Autodesk Fusion 360 part; units mm, degrees
sketch "Sketch1" plane through (0, 0, 0) normal (0, 0, 1) x (1, 0, 0)
  circle A0 centre (18.5, 32.0429) radius 7.5
  circle A1 centre (18.5, -32.0429) radius 7.5
  line L0 (0, 0) -> (80.5902, 0) construction
  line L1 (0, 0) -> (18.5, 32.0429) construction
  arc A2 (14.75, 25.5477) -> (14.75, -25.5477) centre (0, 0) ccw
  arc A3 (13.1121, 37.2602) -> (13.1121, -37.2602) centre (0, 0) ccw
  line L2 (-25.6953, 30) -> (-95.6953, 30)
  line L3 (-95.6953, -30) -> (-25.6953, -30)
  line L4 (0, 0) -> (-230.6084, 0) construction
  circle A4 centre (18.5, 32.0429) radius 3.5
  circle A5 centre (18.5, -32.0429) radius 3.5
  line L5 (-105.6953, 20) -> (-105.6953, -20)
  arc A6 (-95.6953, 30) -> (-105.6953, 20) centre (-95.6953, 20) ccw
  arc A7 (-105.6953, -20) -> (-95.6953, -30) centre (-95.6953, -20) ccw
  circle A8 centre (-95.6953, 20) radius 2.5
  circle A9 centre (-95.6953, -20) radius 2.5
  circle A10 centre (-45.6953, -20) radius 2.5
  circle A11 centre (-45.6953, 20) radius 2.5
  circle A12 centre (-70.6953, 20) radius 2.5
  circle A13 centre (-70.6953, -20) radius 2.5
  point P0 (-105.6953, 30)
  point P1 (-105.6953, -30)
  dimension "d1" = 59
  dimension "d2" = 10
  dimension "d3" = 60
  dimension "d4" = 15
  dimension "d5" = 60
  dimension "d23" = 7
  dimension "d25" = 80
  dimension "d26" = 10
  dimension "d27" = 5
  dimension "d28" = 5
  dimension "d29" = 50
  dimension "d30" = 25
extrude "Extrude1" add sketch "Sketch1" along normal blind 6
fillet "Fillet1" radius 10 4 edges at (13.1121, 37.2602, 3) (-25.6953, 30, 3) (13.1121, -37.2602, 3) (-25.6953, -30, 3)
Can you work these out from the model? Positions are in its coordinate system, mm. Round coordinates to 2 decimals unless told otherwise and drop trailing zeros. Loops run counter-clockwise (first coordinate to the right, second up) from the corner with the lowest first, then second, coordinate; pieces in that order, holes last. Notation, with made-up numbers: M 48,-31 L 78,-31 A21 ccw 78,2 Z; hole C 48.25,-8.5 d2. An arc over 180 degrees is marked long. Answer as a JSON object with one key per item and string values. Group by question number.
Q1. Will this pin go through, and if not, where does the flat tip stop? pin 1 (2 mm diameter, centred on x = 10, z = 2, fed in from -Y).
Q2. We'd pull the mould along X, two halves only. Please class faces 1 (the flat face through (-62, 30, 3)), 2 (the cylindrical face through (25.97, -31.39, 2.96)), 3 (the cylindrical face through (-7.96, 38.69, 2.96)), 4 (the cylindrical face through (-26.019, -30.506, 3.042)): +X half, -X half, draft (parallel to the pull), parting line (faces both ways), or undercut.
Q3. Imagine slicing it at B-B, the plane x = 18.5. Please give me the cut outline in (y, z).
Q4. Imagine slicing it at A-A, the plane x = 0. Please give me the cut outline in (y, z).
Q5. Imagine slicing it at C-C, the plane y = 0. Please give me the cut outline in (x, z), then the cut area to 3 significant figures.
Q6. Please list where these lines run through material, in increasing order: L1, parallel to Y at x = 18.5, z = 4.3; L2, parallel to Y at x = -71, z = 3.5; L3, parallel to Y at x = -65, z = 1.
Q7. Imagine slicing it at D-D, the plane z = 4. Count the separate pieces of the cut face and the enclosed holes in it, then the cut area to 3 significant figures.
Findings:
{
 "1": {"pin 1": "stops at y = -38.46"},
 "2": {"face 1": "draft", "face 2": "undercut", "face 3": "undercut", "face 4": "-X half"},
 "3": {"outline": "M -39.54,0 L -35.54,0 L -35.54,6 L -39.54,6 Z; M -28.54,0 L -24.54,0 L -24.54,6 L -28.54,6 Z; M 24.54,0 L 28.54,0 L 28.54,6 L 24.54,6 Z; M 35.54,0 L 39.54,0 L 39.54,6 L 35.54,6 Z"},
 "4": {"outline": "M -39.5,0 L -29.5,0 L -29.5,6 L -39.5,6 Z; M 29.5,0 L 39.5,0 L 39.5,6 L 29.5,6 Z"},
 "5": {"outline": "M -105.7,0 L -29.5,0 L -29.5,6 L -105.7,6 Z", "area": "457 mm2"},
 "6": {"L1": "y = -39.54 to -35.54, -28.54 to -24.54, 24.54 to 28.54, 35.54 to 39.54", "L2": "y = -30 to -22.48, -17.52 to 17.52, 22.48 to 30", "L3": "y = -30 to 30"},
 "7": {"separate pieces": "1", "enclosed holes": "8", "area": "5,670 mm2"}
}
